Check sheet for the drawn part. Datum: minimum x, y, z corner. Units: mm. Round coordinates to 2 decimals unless told otherwise and drop trailing zeros. Write each loop counter-clockwise with the first axis right and the second up, starting at its lowest first coordinate (ties: lowest second). Pieces come first, ordered by that corner, then holes. Notation, with made-up numbers: M -32,33.5 L -26,33.5 A12 cw -26,41.5 Z; hole C 80,-3 d11. An arc over 180 degrees is marked long. One line per item, written item: value. Start each with the question number.
Item 1: Section check C-C, the plane z = 50.8. Record the cut outline in (x, y).
Item 2: Section check B-B, the plane y = 31. Record the cut outline in (x, z).
Item 3: Section check D-D, the plane y = 52.5. Record the cut outline in (x, z), then the cut area to 3 significant figures.
Item 4: Draft check along Z on the marked faces 1, 2 and 3. Enter one of: +Z half, -Z half, draft (parallel to the pull), parting line (faces both ways), or undercut.
Item 5: Section check A-A, the plane x = 50.8. Record the cut outline in (y, z).
Item 6: Thickness scan on probe 1 along Y at (x, z) = (50, 4); probe 2 along Z at (x, y) = (50, 50); probe 3 along Y at (x, z) = (42, 55). Record the ranges inside material, lowest first. Write a range as from..to.
Item 7: Gauge pin test, flat ends, axial feed: pin 1 (12 mm diameter, centred on y = 31.5, z = 78, fed in from +X); pin 2 (5 mm diameter, centred on y = 37, z = 74, fed in from +X); pin 3 (12 mm diameter, centred on x = 91, z = 66, fed in from +Y); pin 4 (4 mm diameter, centred on x = 37, y = 58, fed in from +Z). Record the tip position at first contact, or that the pin passes through.
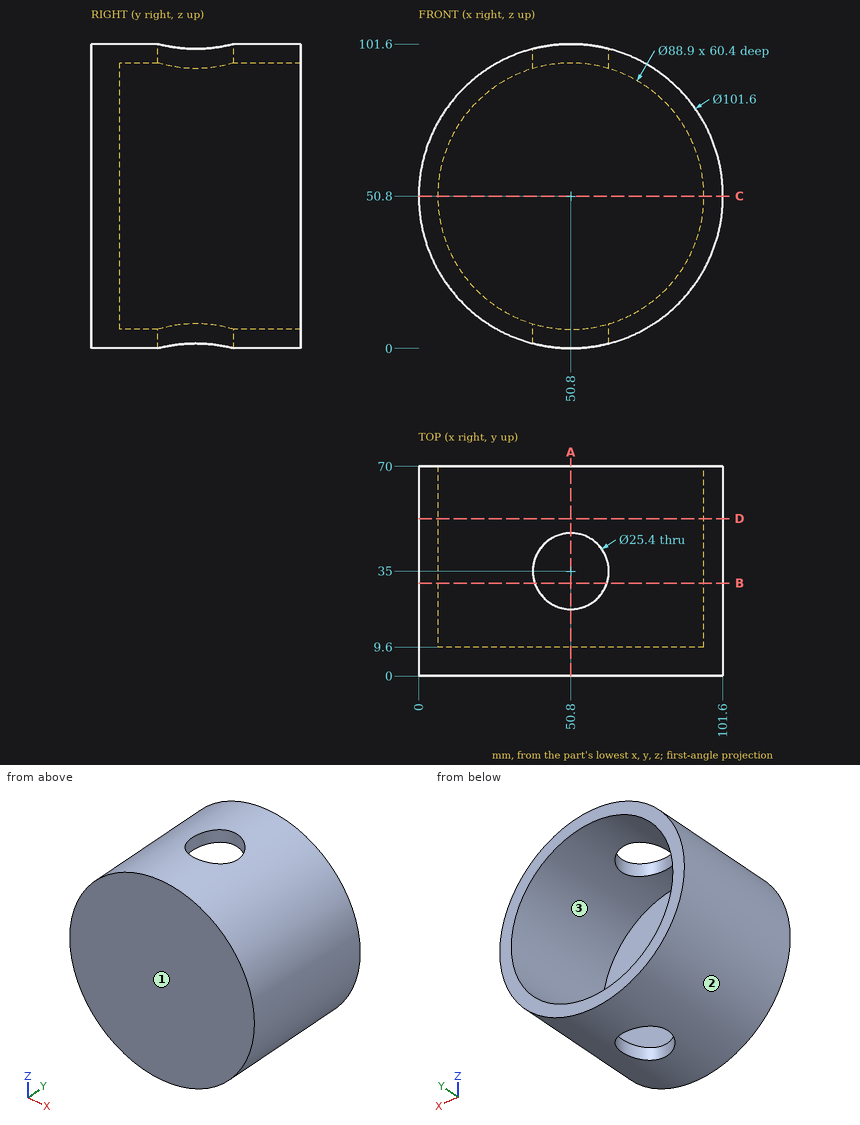
Response values:
1. outline: M 0,0 L 101.6,0 L 101.6,70 L 95.25,70 L 95.25,9.6 L 6.35,9.6 L 6.35,70 L 0,70 Z
2. outline: M 38.75,1.45 L 38.75,8.02 A44.45 cw 38.75,93.58 L 38.75,100.15 A50.8 ccw Z; M 62.85,1.45 A50.8 ccw 62.85,100.15 L 62.85,93.58 A44.45 cw 62.85,8.02 Z
3. outline: C 50.8,50.8 d101.6; hole C 50.8,50.8 d88.9
3. area: 1,900 mm2
4. face 1: draft
4. face 2: parting line
4. face 3: undercut
5. outline: M 0,0 L 22.3,0 L 22.3,6.35 L 9.6,6.35 L 9.6,95.25 L 22.3,95.25 L 22.3,101.6 L 0,101.6 Z; M 47.7,0 L 70,0 L 70,6.35 L 47.7,6.35 Z; M 47.7,95.25 L 70,95.25 L 70,101.6 L 47.7,101.6 Z
6. probe 1: y = 0..22.33, 47.67..70
6. probe 2: z = 0.01..6.36, 95.24..101.59
6. probe 3: y = 0..9.6
7. pin 1: stops at x = 96.96
7. pin 2: stops at x = 97.19
7. pin 3: stops at y = 70
7. pin 4: stops at z = 100.21
